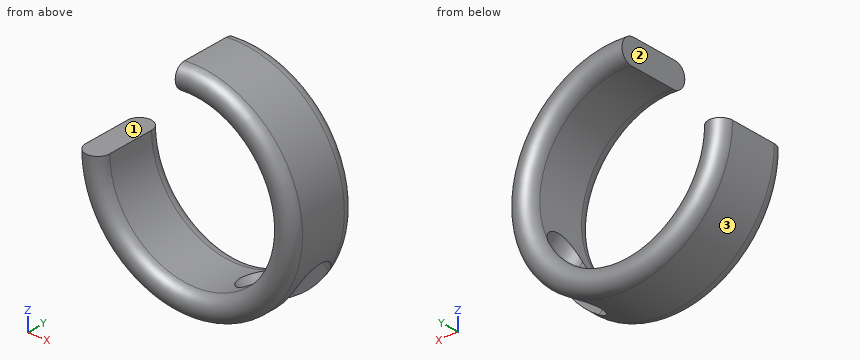
```python
from build123d import *

# Parameters (mm, degrees)
REVOLVE1_ANGLE     = 275
CUT_EXTRUDE1_REACH = 64.273


with BuildPart() as part:
    # Sketch1 → Revolve1 (revolve)
    with BuildSketch(Plane.XY):
        with BuildLine():
            Line((-22.5, -5), (-22.5, 5))
            ThreePointArc((-22.5, 5), (-20, 7.5), (-17.5, 5))
            Line((-17.5, 5), (-17.5, -5))
            ThreePointArc((-17.5, -5), (-20, -7.5), (-22.5, -5))
        make_face()
    revolve(axis=Axis((0, 8.757264849, 0), (0, -1, 0)), revolution_arc=REVOLVE1_ANGLE)

    # Sketch2 → Cut-Extrude1 (cut, up to next)
    with BuildSketch(Plane(origin=(21.213203436, 0, -21.213203436), x_dir=(-0.7071067811865488, 0, -0.7071067811865462), z_dir=(0.7071067811865462, 0, -0.7071067811865488)), mode=Mode.PRIVATE) as cut_extrude1_sk1:
        with BuildLine():
            Line((-5, 5.18337521), (5, 5.18337521))
            ThreePointArc((5, 5.18337521), (9, 1.18337521), (5, -2.81662479))
            Line((5, -2.81662479), (-5, -2.81662479))
            ThreePointArc((-5, -2.81662479), (-9, 1.18337521), (-5, 5.18337521))
        make_face()
    cut_extrude1_tool1 = extrude(cut_extrude1_sk1.sketch, amount=-CUT_EXTRUDE1_REACH, mode=Mode.PRIVATE) & part.part
    add(cut_extrude1_tool1.solids().sort_by_distance((21.213203, 1.183375, -21.213203))[0], mode=Mode.SUBTRACT)


solid = part.part
```
Verification items for the finished model (mm, model axes). Face numbers are marked on the shaded views. Give positions to 0.01 mm unless a question says otherwise; leave off trailing zeros. Loops run counter-clockwise (first coordinate to the right, second up) from the corner with the lowest first, then second, coordinate; pieces in that order, holes last.
1. Thickness scan on line 1 (Z direction, x = 0, y = 0.25); line 2 (Z direction, x = 13, y = 5.5); line 3 (Y direction, x = 12.5, z = -14). Record the ranges inside material, lowest first.
2. Section check C-C, the plane z = -16.5. Count the separate pieces of the cut face and the enclosed holes in it, then the cut area to 3 significant figures.
3. Go/stop test with flat-tipped pins: pin 1 Ø6 at (x, y) = (-18, 5) entering from -Z; pin 2 Ø12 at (x, z) = (-9.5, -6) entering from -Y; pin 3 Ø2 at (x, y) = (-9, -1) entering from -Z; pin 4 Ø5 at (x, y) = (-11, 5.5) entering from +Z. Record where each tip stops, or that it passes through.
4. Section check B-B, the plane y = 1.75. Enter the section's corners in (x, z).
5. Section check A-A, the plane x = 0. Enter the section's corners in (y, z).
6. Section check D-D, the plane y = -4. Enter the section's corners in (x, z), then the cut area to 3 significant figures.
7. Mould release check, pull along Z, two halves, no side actions. Record for the marked faces 1, 2 and 3: released by +Z, released by -Z, zero draft, split by the parting line, or undercut.
Geometry says:
1. line 1: z = -22.5 to -17.5, 17.5 to 22.5
1. line 2: z = -18.3 to -11.79, 11.79 to 18.3
1. line 3: y = -7.18 to -2.82, 5.18 to 7.18
2. separate pieces: 3
2. enclosed holes: 0
2. area: 189 mm2
3. pin 1: stops at z = -16.77
3. pin 2: passes through
3. pin 3: stops at z = -21.03
3. pin 4: stops at z = -11.17
4. outline: (-22.5, 0) arc R22.5 ccw to (8.26, -20.93) - (4.29, -16.96) arc R17.5 cw to (-17.5, 0) - close; (-1.96, 22.41) - (-1.53, 17.43) arc R17.5 cw to (16.96, -4.29) - (20.93, -8.26) arc R22.5 ccw to start
5. outline: (-5, -22.5) - (5, -22.5) arc R2.5 ccw to (5, -17.5) - (-5, -17.5) arc R2.5 ccw to start; (-5, 17.5) - (5, 17.5) arc R2.5 ccw to (5, 22.5) - (-5, 22.5) arc R2.5 ccw to start
6. outline: (-22.5, 0) arc R22.5 ccw (long way) to (-1.96, 22.41) - (-1.53, 17.43) arc R17.5 cw (long way) to (-17.5, 0) - close
6. area: 480 mm2
7. face 1: released by +Z
7. face 2: undercut
7. face 3: split by the parting line
